```python
from build123d import *

# Parameters (mm, degrees)
F1_DEPTH = 1.5


with BuildPart() as f1:
    # F0 (on Top) → F1 (new body)
    with BuildSketch(Plane.XY):
        with BuildLine():
            Line((-58.75, -14.085047), (-58.75, 0))
            Line((-58.75, 0), (-90.75, 0))
            Line((-90.75, 0), (-90.75, -14.085047))
            Line((-90.75, -14.085047), (-90.75, -19.335047))
            ThreePointArc((-90.75, -19.335047), (-89.285534, -22.870581), (-85.75, -24.335047))
            Line((-85.75, -24.335047), (-80.50245, -24.335047))
            Line((-80.50245, -24.335047), (-80.50245, -18.085047))
            Line((-80.50245, -18.085047), (-84.25, -18.085047))
            ThreePointArc((-84.25, -18.085047), (-85.664214, -17.49926), (-86.25, -16.085047))
            ThreePointArc((-86.25, -16.085047), (-85.664214, -14.670833), (-84.25, -14.085047))
            Line((-84.25, -14.085047), (-58.75, -14.085047))
        make_face()
        with BuildLine():
            Line((90.75, 0), (58.75, 0))
            Line((58.75, 0), (51.75, 0))
            Line((51.75, 0), (51.75, -14))
            ThreePointArc((51.75, -14), (51.164214, -15.414214), (49.75, -16))
            Line((49.75, -16), (41.75, -16))
            ThreePointArc((41.75, -16), (40.335786, -15.414214), (39.75, -14))
            Line((39.75, -14), (39.75, 0))
            Line((39.75, 0), (7.5, 0))
            ThreePointArc((7.5, 0), (5.303301, -5.303301), (0, -7.5))
            Line((0, -7.5), (0, -58.75))
            Line((0, -58.75), (20.192911, -58.75))
            ThreePointArc((20.192911, -58.75), (24.019745, -57.988795), (27.263979, -55.821068))
            Line((27.263979, -55.821068), (57.285534, -25.799513))
            ThreePointArc((57.285534, -25.799513), (58.907651, -24.715649), (60.821068, -24.335047))
            Line((60.821068, -24.335047), (85.75, -24.335047))
            ThreePointArc((85.75, -24.335047), (89.285534, -22.870581), (90.75, -19.335047))
            Line((90.75, -19.335047), (90.75, 0))
        make_face()
        with BuildLine():
            Line((58.25, -14.085047), (58.75, -14.085047))
            Line((58.75, -14.085047), (84.25, -14.085047))
            ThreePointArc((84.25, -14.085047), (85.664214, -14.670833), (86.25, -16.085047))
            ThreePointArc((86.25, -16.085047), (85.664214, -17.49926), (84.25, -18.085047))
            Line((84.25, -18.085047), (58.75, -18.085047))
            Line((58.75, -18.085047), (58.25, -18.085047))
            ThreePointArc((58.25, -18.085047), (56.835786, -17.49926), (56.25, -16.085047))
            ThreePointArc((56.25, -16.085047), (56.835786, -14.670833), (58.25, -14.085047))
        make_face(mode=Mode.SUBTRACT)
        with BuildLine():
            Line((51.75, 0), (58.75, 0))
            Line((58.75, 0), (90.75, 0))
            Line((90.75, 0), (90.75, 19.335047))
            ThreePointArc((90.75, 19.335047), (89.285534, 22.870581), (85.75, 24.335047))
            Line((85.75, 24.335047), (60.821068, 24.335047))
            ThreePointArc((60.821068, 24.335047), (58.907651, 24.715649), (57.285534, 25.799513))
            Line((57.285534, 25.799513), (27.263979, 55.821068))
            ThreePointArc((27.263979, 55.821068), (24.019745, 57.988795), (20.192911, 58.75))
            Line((20.192911, 58.75), (0, 58.75))
            Line((0, 58.75), (0, 7.5))
            ThreePointArc((0, 7.5), (5.303301, 5.303301), (7.5, 0))
            Line((7.5, 0), (39.75, 0))
            Line((39.75, 0), (39.75, 14))
            ThreePointArc((39.75, 14), (40.335786, 15.414214), (41.75, 16))
            Line((41.75, 16), (49.75, 16))
            ThreePointArc((49.75, 16), (51.164214, 15.414214), (51.75, 14))
            Line((51.75, 14), (51.75, 0))
        make_face()
        with BuildLine():
            Line((58.25, 18.085047), (58.75, 18.085047))
            Line((58.75, 18.085047), (84.25, 18.085047))
            ThreePointArc((84.25, 18.085047), (85.664214, 17.49926), (86.25, 16.085047))
            ThreePointArc((86.25, 16.085047), (85.664214, 14.670833), (84.25, 14.085047))
            Line((84.25, 14.085047), (58.75, 14.085047))
            Line((58.75, 14.085047), (58.25, 14.085047))
            ThreePointArc((58.25, 14.085047), (56.835786, 14.670833), (56.25, 16.085047))
            ThreePointArc((56.25, 16.085047), (56.835786, 17.49926), (58.25, 18.085047))
        make_face(mode=Mode.SUBTRACT)
        with BuildLine():
            Line((0, -58.75), (0, -7.5))
            ThreePointArc((0, -7.5), (-5.303301, -5.303301), (-7.5, 0))
            Line((-7.5, 0), (-39.75, 0))
            Line((-39.75, 0), (-39.75, -14))
            ThreePointArc((-39.75, -14), (-40.335786, -15.414214), (-41.75, -16))
            Line((-41.75, -16), (-49.75, -16))
            ThreePointArc((-49.75, -16), (-51.164214, -15.414214), (-51.75, -14))
            Line((-51.75, -14), (-51.75, 0))
            Line((-51.75, 0), (-58.75, 0))
            Line((-58.75, 0), (-58.75, -14.085047))
            Line((-58.75, -14.085047), (-58.25, -14.085047))
            ThreePointArc((-58.25, -14.085047), (-56.835786, -14.670833), (-56.25, -16.085047))
            ThreePointArc((-56.25, -16.085047), (-56.835786, -17.49926), (-58.25, -18.085047))
            Line((-58.25, -18.085047), (-58.75, -18.085047))
            Line((-58.75, -18.085047), (-80.50245, -18.085047))
            Line((-80.50245, -18.085047), (-80.50245, -24.335047))
            Line((-80.50245, -24.335047), (-60.821068, -24.335047))
            ThreePointArc((-60.821068, -24.335047), (-58.907651, -24.715649), (-57.285534, -25.799513))
            Line((-57.285534, -25.799513), (-27.263979, -55.821068))
            ThreePointArc((-27.263979, -55.821068), (-24.019745, -57.988795), (-20.192911, -58.75))
            Line((-20.192911, -58.75), (0, -58.75))
        make_face()
        with BuildLine():
            ThreePointArc((-7.5, 0), (-5.303301, 5.303301), (0, 7.5))
            Line((0, 7.5), (0, 58.75))
            Line((0, 58.75), (-20.192911, 58.75))
            ThreePointArc((-20.192911, 58.75), (-24.019745, 57.988795), (-27.263979, 55.821068))
            Line((-27.263979, 55.821068), (-57.285534, 25.799513))
            ThreePointArc((-57.285534, 25.799513), (-58.907651, 24.715649), (-60.821068, 24.335047))
            Line((-60.821068, 24.335047), (-85.75, 24.335047))
            ThreePointArc((-85.75, 24.335047), (-89.285534, 22.870581), (-90.75, 19.335047))
            Line((-90.75, 19.335047), (-90.75, 0))
            Line((-90.75, 0), (-58.75, 0))
            Line((-58.75, 0), (-51.75, 0))
            Line((-51.75, 0), (-51.75, 14))
            ThreePointArc((-51.75, 14), (-51.164214, 15.414214), (-49.75, 16))
            Line((-49.75, 16), (-41.75, 16))
            ThreePointArc((-41.75, 16), (-40.335786, 15.414214), (-39.75, 14))
            Line((-39.75, 14), (-39.75, 0))
            Line((-39.75, 0), (-7.5, 0))
        make_face()
        with BuildLine():
            Line((-58.25, 14.085047), (-58.75, 14.085047))
            Line((-58.75, 14.085047), (-84.25, 14.085047))
            ThreePointArc((-84.25, 14.085047), (-85.664214, 14.670833), (-86.25, 16.085047))
            ThreePointArc((-86.25, 16.085047), (-85.664214, 17.49926), (-84.25, 18.085047))
            Line((-84.25, 18.085047), (-58.75, 18.085047))
            Line((-58.75, 18.085047), (-58.25, 18.085047))
            ThreePointArc((-58.25, 18.085047), (-56.835786, 17.49926), (-56.25, 16.085047))
            ThreePointArc((-56.25, 16.085047), (-56.835786, 14.670833), (-58.25, 14.085047))
        make_face(mode=Mode.SUBTRACT)
    extrude(amount=F1_DEPTH)


solid = f1.part
```
The listing builds one solid part. Answer for the finished solid, in the listing's coordinates (mm). Give positions to 0.01 mm unless a question says otherwise; leave off trailing zeros. Order: outer loops, then holes, each group sorted by start corner. A loop starts at its lowest first (then second) coordinate and runs counter-clockwise, first axis right, second up. Notation, with made-up numbers: M 20,-31 L 72,-31 A27 ccw 72,8 Z; hole C -2.5,6 d5. An arc over 180 degrees is marked long. Put each result on its own line as item: value. Start each with the question number.
Item 1: The part is cut by section C-C, the plane y = 5.5. Determine the outline of the cut face in (x, z).
Item 2: The part is cut by section D-D, the plane x = -5.5. Determine the outline of the cut face in (y, z).
Item 3: The part is cut by section A-A, the plane y = -11.5. Determine the outline of the cut face in (x, z).
Item 4: The part is cut by section B-B, the plane x = -67. Determine the outline of the cut face in (y, z).
Item 5: Find the intervals of material crossed by line 1 along Y through (x, z) = (68, 0.35); line 2 along X through (y, z) = (16.5, 0.4); line 3 along X through (y, z) = (-15.5, 0.35), in increasing order.
Answer key:
1. outline: M -90.75,0 L -51.75,0 L -51.75,1.5 L -90.75,1.5 Z; M -39.75,0 L -5.1,0 L -5.1,1.5 L -39.75,1.5 Z; M 5.1,0 L 39.75,0 L 39.75,1.5 L 5.1,1.5 Z; M 51.75,0 L 90.75,0 L 90.75,1.5 L 51.75,1.5 Z
2. outline: M -58.75,0 L -5.1,0 L -5.1,1.5 L -58.75,1.5 Z; M 5.1,0 L 58.75,0 L 58.75,1.5 L 5.1,1.5 Z
3. outline: M -90.75,0 L -51.75,0 L -51.75,1.5 L -90.75,1.5 Z; M -39.75,0 L 39.75,0 L 39.75,1.5 L -39.75,1.5 Z; M 51.75,0 L 90.75,0 L 90.75,1.5 L 51.75,1.5 Z
4. outline: M -24.34,0 L -18.09,0 L -18.09,1.5 L -24.34,1.5 Z; M -14.09,0 L 14.09,0 L 14.09,1.5 L -14.09,1.5 Z; M 18.09,0 L 24.34,0 L 24.34,1.5 L 18.09,1.5 Z
5. line 1: y = -24.34 to -18.09, -14.09 to 14.09, 18.09 to 24.34
5. line 2: x = -90.75 to -86.21, -56.29 to 56.29, 86.21 to 90.75
5. line 3: x = -90.75 to -86.16, -56.34 to -51.07, -40.43 to 40.43, 51.07 to 56.34, 86.16 to 90.75
